Autodesk Inventor part; units mm, degrees
ref_plane "Work Plane1" through (0, 0, 50.07) normal (0, 0, 1) x (1, 0, 0)
ref_plane "YZ Plane" through (0, 0, 0) normal (1, 0, 0) x (0, 1, 0)
ref_plane "XZ Plane" through (0, 0, 0) normal (0, 1, 0) x (-1, 0, 0)
sketch "Sketch1" plane through (0, 0, 0) normal (0, 0, 1) x (1, 0, 0)
  circle A0 centre (0, 0) radius 3.4
  line L0 (0, 0) -> (20, 20) construction
  line L1 (0, 0) -> (28.2843, 0) construction
  line L2 (20, 20) -> (4.15, 20)
  line L3 (4.15, 20) -> (4.15, 15.5)
  line L4 (4.15, 15.5) -> (7.1, 15.5)
  line L5 (7.1, 15.5) -> (7.1, 18)
  line L6 (7.1, 18) -> (10.25, 18)
  line L7 (10.25, 18) -> (10.25, 14)
  line L8 (0, 0) -> (0, 26.1056) construction
  line L9 (10.25, 14) -> (2.3, 6.05)
  line L10 (2.3, 6.05) -> (0, 6.05)
  circle A1 centre (15, 15) radius 3
  line L11 (20, 20) -> (20, 4.15)
  line L12 (20, 4.15) -> (15.5, 4.15)
  line L13 (15.5, 4.15) -> (15.5, 7.1)
  line L14 (15.5, 7.1) -> (18, 7.1)
  line L15 (18, 7.1) -> (18, 10.25)
  line L16 (18, 10.25) -> (14, 10.25)
  line L17 (14, 10.25) -> (6.05, 2.3)
  line L18 (6.05, 2.3) -> (6.05, 0)
  line L19 (-2.3, 6.05) -> (0, 6.05)
  line L20 (-10.25, 14) -> (-2.3, 6.05)
  line L21 (-10.25, 18) -> (-10.25, 14)
  line L22 (-4.15, 15.5) -> (-7.1, 15.5)
  line L23 (-7.1, 15.5) -> (-7.1, 18)
  line L24 (-7.1, 18) -> (-10.25, 18)
  line L25 (-4.15, 20) -> (-4.15, 15.5)
  line L26 (-20, 20) -> (-4.15, 20)
  circle A2 centre (-15, 15) radius 3
  line L27 (-20, 20) -> (-20, 4.15)
  line L28 (-14, 10.25) -> (-6.05, 2.3)
  line L29 (-18, 7.1) -> (-18, 10.25)
  line L30 (-18, 10.25) -> (-14, 10.25)
  line L31 (-20, 4.15) -> (-15.5, 4.15)
  line L32 (-15.5, 4.15) -> (-15.5, 7.1)
  line L33 (-15.5, 7.1) -> (-18, 7.1)
  line L34 (-6.05, 2.3) -> (-6.05, 0)
  line L35 (-6.05, -2.3) -> (-6.05, 0)
  line L36 (-14, -10.25) -> (-6.05, -2.3)
  line L37 (-18, -10.25) -> (-14, -10.25)
  line L38 (-15.5, -4.15) -> (-15.5, -7.1)
  line L39 (-15.5, -7.1) -> (-18, -7.1)
  line L40 (-18, -7.1) -> (-18, -10.25)
  line L41 (-20, -4.15) -> (-15.5, -4.15)
  line L42 (-20, -20) -> (-20, -4.15)
  circle A3 centre (-15, -15) radius 3
  line L43 (-20, -20) -> (-4.15, -20)
  line L44 (-10.25, -14) -> (-2.3, -6.05)
  line L45 (-7.1, -18) -> (-10.25, -18)
  line L46 (-10.25, -18) -> (-10.25, -14)
  line L47 (-4.15, -20) -> (-4.15, -15.5)
  line L48 (-4.15, -15.5) -> (-7.1, -15.5)
  line L49 (-7.1, -15.5) -> (-7.1, -18)
  line L50 (-2.3, -6.05) -> (0, -6.05)
  line L51 (2.3, -6.05) -> (0, -6.05)
  line L52 (10.25, -14) -> (2.3, -6.05)
  line L53 (10.25, -18) -> (10.25, -14)
  line L54 (4.15, -15.5) -> (7.1, -15.5)
  line L55 (7.1, -15.5) -> (7.1, -18)
  line L56 (7.1, -18) -> (10.25, -18)
  line L57 (4.15, -20) -> (4.15, -15.5)
  line L58 (20, -20) -> (4.15, -20)
  circle A4 centre (15, -15) radius 3
  line L59 (20, -20) -> (20, -4.15)
  line L60 (14, -10.25) -> (6.05, -2.3)
  line L61 (18, -7.1) -> (18, -10.25)
  line L62 (18, -10.25) -> (14, -10.25)
  line L63 (20, -4.15) -> (15.5, -4.15)
  line L64 (15.5, -4.15) -> (15.5, -7.1)
  line L65 (15.5, -7.1) -> (18, -7.1)
  line L66 (6.05, -2.3) -> (6.05, 0)
  point P0 (0, 6.05)
  point P1 (-6.05, 0)
  point P2 (0, -6.05)
  dimension "d0" = 6.8
  dimension "d1" = 45
  dimension "d2" = 20
  dimension "d3" = 6
  dimension "d4" = 15
  dimension "d5" = 10.25
  dimension "d6" = 7.1
  dimension "d7" = 4.15
  dimension "d8" = 4.5
  dimension "d9" = 2
  dimension "d10" = 13.95
  dimension "d11" = 6
  dimension "d14" = 360
extrude "Extrusion1" add sketch "Sketch1" along normal blind 100.14
ref_plane "Work Plane1" through (0, 0, 50.07) normal (0, 0, 1) x (1, 0, 0)
properties part number "Aluminum_Profile_4040_100.14mm_bottom" material "Aluminum 6061-AHC"
Input: part model. Units: mm. Frame: model coordinates. A direction names the side the tool comes from. Coordinates: 2 decimals unless noted, no trailing zeros. Loops run counter-clockwise (first coordinate to the right, second up) from the corner with the lowest first, then second, coordinate; pieces in that order, holes last. Notation, with made-up numbers: M 57,24 L 75,24 A19 ccw 75,40 Z; hole C 88.5,56.25 d2. An arc over 180 degrees is marked long. Answer in a Markdown table with one row per item.
1. Material intervals for line 1 (Y direction, x = -15, z = 44.5); line 2 (Y direction, x = -7, z = 27); line 3 (X direction, y = 10, z = 72), sorted ascending.
Response:
| item | result |
|---|---|
| line 1 | y = -20 to -18, -12 to -10.25, 10.25 to 12, 18 to 20 |
| line 2 | y = -20 to -15.5, -10.75 to -3.25, 3.25 to 10.75, 15.5 to 20 |
| line 3 | x = -20 to -18, -13.75 to -6.25, 6.25 to 13.75, 18 to 20 |
2. Reachability of faces 1 (the flat face through (-18, -4.15, 49)), 2 (the flat face through (6.05, 0, 49)), 3 (the flat face through (4.15, 18, 49)), 4 (the flat face through (-16, -10.25, 49)) from +Z, -Z, +X, -X, +Y, -Y: full face, straight path, thin tool, end or side. Return the list, or none.
Response:
| item | result |
|---|---|
| face 1 | +Z, -Z, -X |
| face 2 | +Z, -Z, +X |
| face 3 | +Z, -Z, +Y |
| face 4 | +Z, -Z |
3. First-contact query: pin 1 (8 mm diameter, centred on x = -15.5, y = -15.5, fed in from +Z); pin 2 (5.5 mm diameter, centred on x = -15, y = -15, fed in from -Z); pin 3 (5 mm diameter, centred on x = 0, z = 63.5, fed in from -Y). Flat tips, straight axial feed; report the tip coordinate or a pass-through.
Response:
| item | result |
|---|---|
| pin 1 | stops at z = 100.14 |
| pin 2 | passes through |
| pin 3 | stops at y = -6.25 |
4. Section C-C, the plane z = 55.5. Count the separate pieces of the cut face and the enclosed holes in it, then the cut area to 3 significant figures.
Response:
| item | result |
|---|---|
| separate pieces | 1 |
| enclosed holes | 5 |
| area | 716 mm2 |
5. Draft query along Y for faces 5 (the flat face through (-10.08, -6.33, 49.37)), 6 (the flat face through (-4.15, -18, 49)), 7 (the flat face through (-12, -20, 49)). Return one class per face: pulls with the +Y half, pulls with the -Y half, needs draft (parallel to the pull), parting line crosses it, or undercut.
Response:
| item | result |
|---|---|
| face 5 | undercut |
| face 6 | needs draft |
| face 7 | pulls with the -Y half |
6. Section A-A, the plane y = 0. Output: boundary loops of the cut face in (x, z).
Response:
| item | result |
|---|---|
| outline | M -6.05,0 L -3.4,0 L -3.4,100.14 L -6.05,100.14 Z; M 3.4,0 L 6.05,0 L 6.05,100.14 L 3.4,100.14 Z |
